```python
from build123d import *

# Parameters (mm, degrees)
F1_DEPTH  = 6.9
F2_R      = 1.5
F3_DEPTH  = 16.6
F4_W      = 13.5
F4_H      = 22.5
F5_DEPTH  = 5.75
F6_R      = 1.75
F7_DEPTH  = 0.5
F8_R      = 0.75
F9_DEPTH  = 4.5
F10_W     = 0.3
F10_H     = 2.5
F11_DEPTH = 4


with BuildPart() as f1:
    # F0 (on Top) → F1 (new body, symmetric)
    with BuildSketch(Plane.XY):
        with BuildLine():
            ThreePointArc((0, -10), (7.071068, -7.071068), (10, 0))
            ThreePointArc((10, 0), (7.071068, 7.071068), (0, 10))
            ThreePointArc((0, 10), (-10, 0), (0, -10))
        make_face()
        with BuildLine():
            ThreePointArc((0, 10), (7.071068, 7.071068), (10, 0))
            ThreePointArc((10, 0), (7.071068, -7.071068), (0, -10))
            Line((0, -10), (26.1, -10))
            Line((26.1, -10), (28.5, -12.4))
            Line((28.5, -12.4), (31.5, -12.4))
            Line((31.5, -12.4), (31.5, 0))
            Line((31.5, 0), (31.5, 12.4))
            Line((31.5, 12.4), (28.5, 12.4))
            Line((28.5, 12.4), (26.1, 10))
            Line((26.1, 10), (0, 10))
        make_face()
    extrude(amount=F1_DEPTH, both=True)

    # F2 (on Top) → F3 (join)
    with BuildSketch(Plane.XY):
        Circle(F2_R)
    extrude(amount=F3_DEPTH)

    # F4 (on Top) → F5 (join, symmetric)
    with BuildSketch(Plane.XY):
        with Locations((38.25, 0)):
            Rectangle(F4_W, F4_H)
    extrude(amount=F5_DEPTH, both=True)

    # F6 (on face) → F7 (join)
    with BuildSketch(Plane.YZ.offset(45)):
        Circle(F6_R)
    extrude(amount=F7_DEPTH)

    # F8 (on face) → F9 (join)
    with BuildSketch(Plane.YZ.offset(45.5)):
        Circle(F8_R)
    extrude(amount=F9_DEPTH)

    # F10 (on face) → F11 (join)
    with BuildSketch(Plane.YZ.offset(45)):
        with Locations((-6.75, 0)):
            Rectangle(F10_W, F10_H)
        with Locations((6.75, 0)):
            Rectangle(F10_W, F10_H)
    extrude(amount=F11_DEPTH)


solid = f1.part
```
Verification items for the finished model (mm, model axes). A direction names the side the tool comes from. Coordinates: 2 decimals unless noted, no trailing zeros. Order: outer loops, then holes, each group sorted by start corner. A loop starts at its lowest first (then second) coordinate and runs counter-clockwise, first axis right, second up. Notation, with made-up numbers: (3, -9.75) -> (61, -9.75) arc R16 cw to (61, 2.25) -> close; hole circle Ø4 at (33, 7.25). An arc over 180 degrees is marked (long way). Answer as CSV lines item,"result". Start each with the question number.
1) Cross-section at B-B, the plane y = 0. Record the boundary of the cut face in (x, z), then the cut area to 3 significant figures.
2) Cross-section at D-D, the plane y = -2.75. Record the boundary of the cut face in (x, z), then the cut area to 3 significant figures.
3) Release check for a two-part mould opening along Y. For faces 1 (the face through (13, 10, 0)), 2 (the face through (47, 6.6, 0)), 3 (the face through (47, -6.9, 0)) record: released by +Y, released by -Y, zero draft, split by the parting line, or undercut.
4) Cross-section at C-C, the plane x = 39. Record the boundary of the cut face in (y, z).
5) Cross-section at A-A, the plane z = 0. Record the boundary of the cut face in (x, y).
6) Set-up check for faces 4 (the face through (-1.5, 0.07, 11.68)), 5 (the face through (47, 6.9, 0)), 6 (the face through (47.72, -0.75, 0.03)): record each of +Z, -Z, +X, -X, +Y, -Y from which the full face is reachable in a straight line by a thin tool's end or side.
7) Gauge pin test, flat ends, axial feed: pin 1 Ø1.5 at (y, z) = (10, 2) entering from +X; pin 2 Ø1 at (x, z) = (20.5, -0.5) entering from -Y; pin 3 Ø2 at (x, z) = (47, 0.5) entering from +Y. Record the tip position at first contact, or that the pin passes through.
8) Material ranges on L1, parallel to Y at x = 7, z = 6; L2, parallel to Z at x = 14, y = 1.75; L3, parallel to Z at x = 42.5, y = -1.25, recorded low to high. Write a range as [from, to].
Conclusion:
1,outline,"(-10, -6.9) -> (31.5, -6.9) -> (31.5, -5.75) -> (45, -5.75) -> (45, -1.75) -> (45.5, -1.75) -> (45.5, -0.75) -> (50, -0.75) -> (50, 0.75) -> (45.5, 0.75) -> (45.5, 1.75) -> (45, 1.75) -> (45, 5.75) -> (31.5, 5.75) -> (31.5, 6.9) -> (1.5, 6.9) -> (1.5, 16.6) -> (-1.5, 16.6) -> (-1.5, 6.9) -> (-10, 6.9) -> close"
1,area,"766 mm²"
2,outline,"(-9.61, -6.9) -> (31.5, -6.9) -> (31.5, -5.75) -> (45, -5.75) -> (45, 5.75) -> (31.5, 5.75) -> (31.5, 6.9) -> (-9.61, 6.9) -> close"
2,area,"723 mm²"
3,face 1,"released by +Y"
3,face 2,"undercut"
3,face 3,"released by -Y"
4,outline,"(-11.25, -5.75) -> (11.25, -5.75) -> (11.25, 5.75) -> (-11.25, 5.75) -> close"
5,outline,"(0, -10) -> (26.1, -10) -> (28.5, -12.4) -> (31.5, -12.4) -> (31.5, -11.25) -> (45, -11.25) -> (45, -6.9) -> (49, -6.9) -> (49, -6.6) -> (45, -6.6) -> (45, -1.75) -> (45.5, -1.75) -> (45.5, -0.75) -> (50, -0.75) -> (50, 0.75) -> (45.5, 0.75) -> (45.5, 1.75) -> (45, 1.75) -> (45, 6.6) -> (49, 6.6) -> (49, 6.9) -> (45, 6.9) -> (45, 11.25) -> (31.5, 11.25) -> (31.5, 12.4) -> (28.5, 12.4) -> (26.1, 10) -> (0, 10) arc R10 ccw to start"
6,face 4,"+Z"
6,face 5,"+Z, -Z, +X, +Y"
6,face 6,"+X"
7,pin 1,"stops at x = 45"
7,pin 2,"stops at y = -10"
7,pin 3,"stops at y = 6.9"
8,L1,"y = [-10, 10]"
8,L2,"z = [-6.9, 6.9]"
8,L3,"z = [-5.75, 5.75]"
